Here's how the part is built. I have some questions about the finished solid (model axes, mm). A direction names the side the tool comes from. Round coordinates to 2 decimals unless told otherwise and drop trailing zeros. Loops run counter-clockwise (first coordinate to the right, second up) from the corner with the lowest first, then second, coordinate; pieces in that order, holes last. Notation, with made-up numbers: M 36,29 L 84,29 A28 ccw 84,48 Z; hole C 74.25,-30.5 d6. An arc over 180 degrees is marked long. Answer as a JSON object with one key per item and string values.
from build123d import *

# Parameters (mm, degrees)
SKETCH1_W           = 105
SKETCH1_H           = 10
SKETCH1_R           = 1.5
BOSS_EXTRUDE1_DEPTH = 3
SKETCH2_W           = 10.5
SKETCH2_H           = 3
CUT_EXTRUDE1_DEPTH  = 53.82281704
SKETCH3_R           = 2
CUT_EXTRUDE3_DEPTH  = 10


with BuildPart() as part:
    # Sketch1 → Boss-Extrude1 (new body)
    with BuildSketch(Plane(origin=(0, 0, 0), x_dir=(1, 0, 0), z_dir=(0, 1, 0))):
        Rectangle(SKETCH1_W, SKETCH1_H)
        with Locations(Location((0, 0, 0), (0, 0, 270))):
            Circle(SKETCH1_R, mode=Mode.SUBTRACT)
    extrude(amount=BOSS_EXTRUDE1_DEPTH)

    # Sketch2 → Cut-Extrude1 (cut, through all)
    with BuildSketch(Plane(origin=(0, 3, 0), x_dir=(1, 0, 0), z_dir=(0, 1, 0))):
        with Locations((-47.25, -3.5)):
            Rectangle(SKETCH2_W, SKETCH2_H)
    cut_extrude1 = extrude(amount=-CUT_EXTRUDE1_DEPTH, mode=Mode.SUBTRACT)

    # Mirror2: Cut-Extrude1 across plane
    add(cut_extrude1.mirror(Plane(origin=(0, 0, 0), x_dir=(0, 0, 1), z_dir=(1, 0, 0))), mode=Mode.SUBTRACT)

    # Sketch3 → Cut-Extrude3 (cut)
    with BuildSketch(Plane.XZ):
        with Locations(Location((-35, -2, 0), (0, 0, 270))):
            Circle(SKETCH3_R)
    extrude(amount=-CUT_EXTRUDE3_DEPTH, mode=Mode.SUBTRACT)


solid = part.part
Item 1: I want a section at C-C, the plane y = 1.85. Please give me the cut outline in (x, z).
Resolved:
{"outline": "M -52.5,-5 L 52.5,-5 L 52.5,2 L 42,2 L 42,5 L -42,5 L -42,2 L -52.5,2 Z; hole C -35,-2 d4; hole C 0,0 d3"}
Item 2: I want a section at B-B, the plane z = -2.75. Please give me the cut outline in (x, y).
Resolved:
{"outline": "M -52.5,0 L -36.85,0 L -36.85,3 L -52.5,3 Z; M -33.15,0 L 52.5,0 L 52.5,3 L -33.15,3 Z"}
Item 3: I want a section at A-A, the plane x = -35. Please give me the cut outline in (y, z).
Resolved:
{"outline": "M 0,-5 L 3,-5 L 3,-4 L 0,-4 Z; M 0,0 L 3,0 L 3,5 L 0,5 Z"}
Item 4: I'm going to push flat-ended pins straight in: pin 1 Ø1.5 at (y, z) = (2, 4) entering from +X; pin 2 Ø5 at (x, z) = (0, 0) entering from +Y; pin 3 Ø1.5 at (y, z) = (1.5, 3.5) entering from -X; pin 4 Ø1.5 at (x, y) = (46.5, 2) entering from +Z. Where does each tip first touch, or does it pass through?
Resolved:
{"pin 1": "x = 42", "pin 2": "y = 3", "pin 3": "x = -42", "pin 4": "z = 2"}
Item 5: On a 3-axis mill with a long thin cutter (end or side, diameter ignored), from which of +Z, -Z, +X, -X, +Y, -Y can I reach the whole of each face in a straight line? I mean faces 1 (the face through (0.45, 1.48, 1.43)), 2 (the face through (-47, 2, 2)), 3 (the face through (47, 2, 2)). Say none if no direction works.
Resolved:
{"face 1": "+Y, -Y", "face 2": "+Z, -X, +Y, -Y", "face 3": "+Z, +X, +Y, -Y"}
Item 6: Please list where these lines run through material, in increasing order: probe 1 along X at (y, z) = (2.45, -2); probe 2 along X at (y, z) = (2.25, 3); probe 3 along Z at (x, y) = (-47.5, 0.4). Write a range as from..to.
Resolved:
{"probe 1": "-52.5..-37, -33..52.5", "probe 2": "-42..42", "probe 3": "-5..2"}
Item 7: If we mould it in two halves opening along X, with no side actions, what happens to faces 4 (the face through (-37, 1, -2)), 5 (the face through (-1, 3, -2)), 6 (the face through (-42, 2, 4))? For each: pulls with the +X half, pulls with the -X half, needs draft (parallel to the pull), parting line crosses it, or undercut.
Resolved:
{"face 4": "undercut", "face 5": "needs draft", "face 6": "pulls with the -X half"}
